Design review of the part built by this model. Coordinates are the model's own, in mm. Give positions to 0.01 mm unless a question says otherwise; leave off trailing zeros. Loops run counter-clockwise (first coordinate to the right, second up) from the corner with the lowest first, then second, coordinate; pieces in that order, holes last. Notation, with made-up numbers: M 48,73 L 75,73 A19 ccw 75,79 Z; hole C -10,88.25 d9. An arc over 180 degrees is marked long. Use one line per item in the form item = value. Start each with the question number.
Autodesk Inventor part; units mm, degrees
ref_plane "YZ Plane" through (0, 0, 0) normal (1, 0, 0) x (0, 1, 0)
ref_plane "XZ Plane" through (0, 0, 0) normal (0, 1, 0) x (-1, 0, 0)
ref_plane "XY Plane" through (0, 0, 0) normal (0, 0, 1) x (1, 0, 0)
sketch "Szkic1" plane through (0, 0, 0) normal (0, 0, 1) x (1, 0, 0)
  circle A0 centre (0, 0) radius 6
  circle A1 centre (0, 0) radius 2.5
  dimension "d0" = 12
  dimension "d1" = 5
extrude "Wyciągnięcie proste1" add sketch "Szkic1" along normal blind 5
chamfer "Faza1" distance 0.3 angle 45 2 edges at (-6, 0, 5) (-6, 0, 0)
chamfer "Faza2" distance 0.3 angle 45 2 edges at (-2.5, 0, 5) (-2.5, 0, 0)
properties part number "COTS_GENERIC_Bearing_12x5x5"
Q1. Take a section at C-C on z = 4.2. Give the boundary of the cut face in (x, y).
Q2. Clearance check with flat-ended pins moving along their axes: pin 1 Ø1 at (x, z) = (-4, 1.5) entering from -Y; pin 2 Ø2 at (y, z) = (-3.5, 2) entering from -X. State where each tip first meets the part, or that it passes through.
Q3. Wall thickness on probe 1 along Y at (x, z) = (0, 1.4); probe 2 along Y at (x, z) = (2, 1.7); probe 3 along Y at (x, z) = (-4, 1.45): over which ranges is each line inside the solid? List them lowest first.
Q4. Take a section at A-A on y = 0. Give the boundary of the cut face in (x, z).
Q5. The part is to be moulded in two halves that separate along Y. For faces 1 (the cylindrical face through (-0.54, 2.44, 2.47)), 2 (the cylindrical face through (-6, 0, 2)), 3 (the flat face through (-3, -1, 5)), say which applies: pulls with the +Y half, pulls with the -Y half, needs draft (parallel to the pull), parting line crosses it, or undercut.
Response values:
q1.outline = C 0,0 d12; hole C 0,0 d5
q2.pin_1 = -4.87
q2.pin_2 = -5.45
q3.probe_1 = -6 to -2.5, 2.5 to 6
q3.probe_2 = -5.66 to -1.5, 1.5 to 5.66
q3.probe_3 = -4.47 to 4.47
q4.outline = M -6,0.3 L -5.7,0 L -2.8,0 L -2.5,0.3 L -2.5,4.7 L -2.8,5 L -5.7,5 L -6,4.7 Z; M 2.5,0.3 L 2.8,0 L 5.7,0 L 6,0.3 L 6,4.7 L 5.7,5 L 2.8,5 L 2.5,4.7 Z
q5.face_1 = undercut
q5.face_2 = parting line crosses it
q5.face_3 = needs draft
